Geometry: see drawing. Coordinates: mm, zero at the bounding-box minimum. A direction names the side the tool comes from. Coordinates: 2 decimals unless noted, no trailing zeros. Loops run counter-clockwise (first coordinate to the right, second up) from the corner with the lowest first, then second, coordinate; pieces in that order, holes last. Notation, with made-up numbers: (-20.5, 13.5) - (18.5, 13.5) arc R28 ccw to (18.5, 49.5) - close; hole circle Ø11 at (60, 40.25). An arc over 180 degrees is marked (long way). Use one line per item in the form item = value.
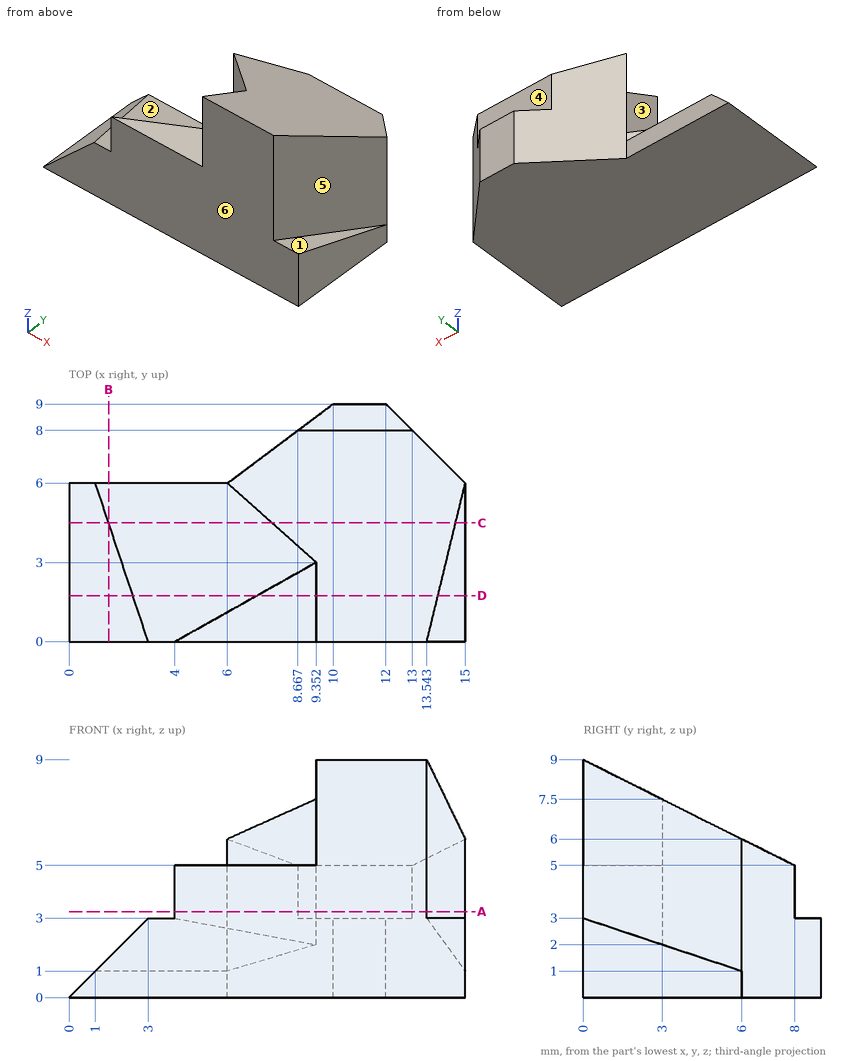
Q1. Cut plane B-B, the plane x = 1.5. Return loops of the section in (y, z).
Check values:
outline = (0, 0) - (6, 0) - (6, 1) - (4.5, 1.5) - (0, 1.5) - close
Q2. First-contact query: P1, Ø3.5, axis at x = 6.5, y = 1.5, coming from the +Z side; P2, Ø2, axis at y = 2, z = 4, coming from the +X side; P3, Ø0.5, axis at x = 2, z = 0.5, coming from the +Y side. Flat tips, straight axial feed; report the tip coordinate or a pass-through.
Check values:
P1 = 5
P2 = 14.27
P3 = 6
Q3. Pull-direction query (Y, two-part tool) for the marked faces 4, 5 and 6; classes: pulls with the +Y half, pulls with the -Y half, needs draft (parallel to the pull), parting line crosses it, or undercut.
Check values:
face_4 = pulls with the +Y half
face_5 = undercut
face_6 = pulls with the -Y half
Q4. Cut plane D-D, the plane y = 1.75. Return loops of the section in (x, z) (1 decimal).
Check values:
outline = (0, 0) - (15, 0) - (15, 2.4) - (14, 2.4) - (14, 8.1) - (9.4, 8.1) - (9.4, 5) - (7.1, 5) - (7.1, 2.4) - (2.4, 2.4) - close
Q5. Ray query, line 1 along Z through (x, y) = (10.25, 8.75); line 2 along Y through (x, z) = (10, 8). Return the intervals inside material, ascending. Write a range as [from, to].
Check values:
line_1 = [0, 3]
line_2 = [0, 2]
Q6. Cut plane A-A, the plane z = 3.25. Return loops of the section in (x, y).
Check values:
outline = (4, 0) - (13.54, 0) - (15, 6) - (13, 8) - (8.67, 8) - (6, 6) - (9.35, 3) - close
Q7. Set-up query: the marked faces 1, 2 and 3. Return all of +Z, -Z, +X, -X, +Y, -Y with unobstructed straight access to the full face (end or side cutting, diameter ignored); none if empty.
Check values:
face_1 = +Z, +X
face_2 = +Z, -X
face_3 = +Z, -X, -Y
Q8. Cut plane C-C, the plane y = 4.5. Return loops of the section in (x, z).
Check values:
outline = (0, 0) - (15, 0) - (15, 1.5) - (14.64, 1.5) - (14.64, 6.75) - (7.68, 6.75) - (7.68, 1.5) - (1.5, 1.5) - close
